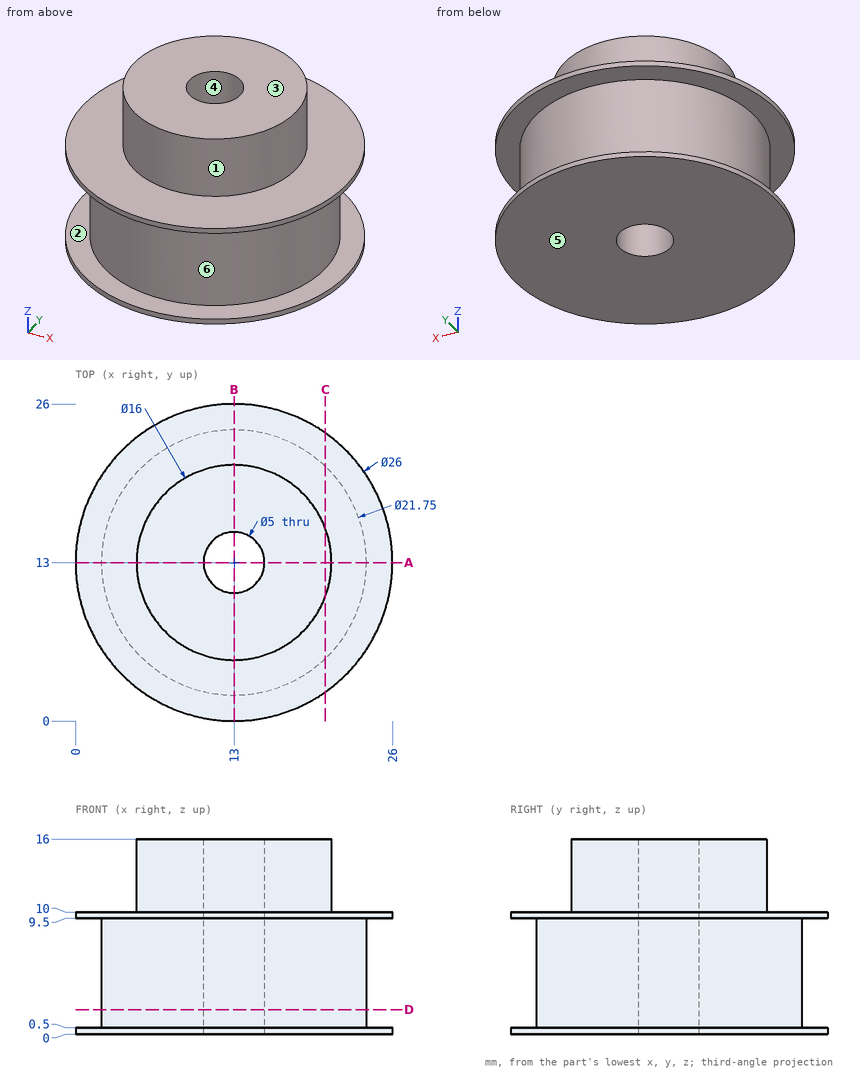
Design review of the part shown in the three views and the two pictorial views. Dimensions are in mm from the part's minimum x, y and z. A direction names the side the tool comes from. Coordinates: 2 decimals unless noted, no trailing zeros. Order: outer loops, then holes, each group sorted by start corner. A loop starts at its lowest first (then second) coordinate and runs counter-clockwise, first axis right, second up. Notation, with made-up numbers: (61.25, 11.5) - (102.25, 11.5) arc R34 cw to (102.25, 46.5) - close; hole circle Ø2 at (42, 78.5). An arc over 180 degrees is marked (long way). Answer as CSV lines item,"result". Start each with the question number.
1) To check wall thickness, follow line 1 along Y through (x, z) = (13, 9.25) (3 decimals); line 2 along Z through (x, y) = (19.25, 22.5); line 3 along Y through (x, z) = (13, 10.75). State the ranges of each line that lie inside material, in increasing order. Write a range as [from, to].
2) Add section D-D (z = 2). State the section outline as (x, y) points (3 decimals), then the cut area to 3 significant figures.
3) Machinability: for the marked faces 1, 2 and 3, which of the approach directions +Z, -Z, +X, -X, +Y, -Y give a long, thin tool a straight path to every point of the face, cutting with its end or side? Answer none if there is none.
4) Insertion check: P1, Ø4, axis at y = 6.5, z = 10.5, coming from the -X side; P2, Ø1.5, axis at x = 21.5, z = 4.5, coming from the -Y side; P3, Ø1, axis at y = 13.5, z = 4.5, coming from the +X side (3 decimals). Each pin has a flat end and moves straight along its axis. Give the tip position at first contact, or say it passes through.
5) Add section C-C (x = 20.5). State the section outline as (y, z) points (3 decimals).
6) Draft analysis for pull direction X (two halves, no side actions). For the marked faces 4, 5 and 6, state which applies: +X half, -X half, draft (parallel to the pull), parting line (faces both ways), or undercut.
7) Add section A-A (y = 13). State the section outline as (x, z) points (3 decimals).
Result:
1,line 1,"[2.125, 10.5], [15.5, 23.875]"
1,line 2,"[0, 0.5], [9.5, 10]"
1,line 3,"[5, 10.5], [15.5, 21]"
2,outline,"circle Ø21.75 at (13, 13); hole circle Ø5 at (13, 13)"
2,area,"352 mm^2"
3,face 1,"+Z"
3,face 2,"none"
3,face 3,"+Z, +X, -X, +Y, -Y"
4,P1,"x = 0.83"
4,P2,"y = 5.37"
4,P3,"x = 23.875"
5,outline,"(2.382, 0) - (23.618, 0) - (23.618, 0.5) - (20.875, 0.5) - (20.875, 9.5) - (23.618, 9.5) - (23.618, 10) - (15.784, 10) - (15.784, 16) - (10.216, 16) - (10.216, 10) - (2.382, 10) - (2.382, 9.5) - (5.125, 9.5) - (5.125, 0.5) - (2.382, 0.5) - close"
6,face 4,"undercut"
6,face 5,"draft"
6,face 6,"parting line"
7,outline,"(0, 0) - (10.5, 0) - (10.5, 16) - (5, 16) - (5, 10) - (0, 10) - (0, 9.5) - (2.125, 9.5) - (2.125, 0.5) - (0, 0.5) - close; (15.5, 0) - (26, 0) - (26, 0.5) - (23.875, 0.5) - (23.875, 9.5) - (26, 9.5) - (26, 10) - (21, 10) - (21, 16) - (15.5, 16) - close"
